Input: part model. Units: mm. Frame: model coordinates. A direction names the side the tool comes from. Coordinates: 2 decimals unless noted, no trailing zeros. Loops run counter-clockwise (first coordinate to the right, second up) from the corner with the lowest first, then second, coordinate; pieces in that order, holes last. Notation, with made-up numbers: (34.25, -23.5) -> (77.25, -23.5) arc R20 ccw to (77.25, 14.5) -> close; hole circle Ø9 at (9.25, -18). An arc over 180 degrees is marked (long way). Put each result on its own line as item: value. Start each with the question number.
1) Cut plane B-B (x = 0). Return the cut outline in (y, z), plus the area to 3 significant figures.
2) Cut plane C-C (y = 1.75). Return the cut outline in (x, z).
3) Cut plane A-A (z = 10). Return the cut outline in (x, y), plus the area to 3 significant figures.
4) Set-up query: faces 1 (the flat face through (2, -4, 20)), 2 (the flat face through (-8, -4, 10)). Return all of +Z, -Z, +X, -X, +Y, -Y with unobstructed straight access to the full face (end or side cutting, diameter ignored); none if empty.
5) Contact query for flat-ended pins moving along their axis: P1, Ø2.5, axis at y = -2, z = 7.5, coming from the +X side; P2, Ø5, axis at x = 0, y = 0, coming from the +Z side; P3, Ø6, axis at x = 14, z = 3, coming from the +Y side; P4, Ø5, axis at y = -1, z = 7, coming from the -X side. Output: stop coordinate, or through.
6) Material intervals for L1, parallel to Y at x = -11.5, z = 2; L2, parallel to Y at x = 0, z = 6.25; L3, parallel to X at y = -2.25, z = 1.5, sorted ascending.
7) Cut plane D-D (z = 4.25). Return the cut outline in (x, y).
8) Pull-direction query (Y, two-part tool) for faces 3 (the flat face through (8, -4, 10)), 4 (the flat face through (13, -8, 12)), 5 (the cylindrical face through (-0.534, 4.065, 9.86)); classes: pulls with the +Y half, pulls with the -Y half, needs draft (parallel to the pull), parting line crosses it, or undercut.
from build123d import *

# Parameters (mm, degrees)
ESBO_O1_R                = 4.1
RESSALTO_EXTRUS_O1_DEPTH = 20
ESBO_O2_R                = 1.6
CORTE_EXTRUS_O1_DEPTH    = 20
FILETE1_R                = 7


with BuildPart() as part:
    # Esboço1 → Ressalto-extrusão1 (new body)
    with BuildSketch(Plane.XY):
        with BuildLine():
            Line((-8, 0), (-8, -8))
            Line((-8, -8), (-18, -8))
            Line((-18, -8), (-18, -12))
            Line((-18, -12), (18, -12))
            Line((18, -12), (18, -8))
            Line((18, -8), (8, -8))
            Line((8, -8), (8, 0))
            ThreePointArc((8, 0), (0, 8), (-8, 0))
        make_face()
        Circle(ESBO_O1_R, mode=Mode.SUBTRACT)
    extrude(amount=RESSALTO_EXTRUS_O1_DEPTH)

    # Esboço2 → Corte-extrusão1 (cut)
    with BuildSketch(Plane(origin=(0, -8, 0), x_dir=(1, 0, 0), z_dir=(0, 1, 0))):
        with Locations(Location((-12.5, -10, 0), (0, 0, 180))):
            Circle(ESBO_O2_R)
        with Locations(Location((12.5, -10, 0), (0, 0, 180))):
            Circle(ESBO_O2_R)
    extrude(amount=-CORTE_EXTRUS_O1_DEPTH, mode=Mode.SUBTRACT)

    # Filete1
    filete1_edges = [part.edges().sort_by_distance(p)[0] for p in [
        (-18, -10, 20),
        (18, -10, 20),
        (18, -10, 0),
        (-18, -10, 0),
    ]]
    fillet(filete1_edges, radius=FILETE1_R)


solid = part.part
Results found:
1. outline: (-12, 0) -> (-4.1, 0) -> (-4.1, 20) -> (-12, 20) -> close; (4.1, 0) -> (8, 0) -> (8, 20) -> (4.1, 20) -> close
1. area: 236 mm2
2. outline: (-7.81, 0) -> (-3.71, 0) -> (-3.71, 20) -> (-7.81, 20) -> close; (3.71, 0) -> (7.81, 0) -> (7.81, 20) -> (3.71, 20) -> close
3. outline: (-18, -12) -> (-14.1, -12) -> (-14.1, -8) -> (-18, -8) -> close; (-10.9, -12) -> (10.9, -12) -> (10.9, -8) -> (8, -8) -> (8, 0) arc R8 ccw to (-8, 0) -> (-8, -8) -> (-10.9, -8) -> close; (14.1, -12) -> (18, -12) -> (18, -8) -> (14.1, -8) -> close; hole circle Ø8.2 at (0, 0)
3. area: 294 mm2
4. face 1: +Z, +X, -X, +Y, -Y
4. face 2: +Z, -Z, -X, +Y
5. P1: stops at x = 8
5. P2: passes through
5. P3: stops at y = -8
5. P4: stops at x = -8
6. L1: y = -12 to -8
6. L2: y = -12 to -4.1, 4.1 to 8
6. L3: x = -8 to -3.43, 3.43 to 8
7. outline: (-17.44, -12) -> (17.44, -12) -> (17.44, -8) -> (8, -8) -> (8, 0) arc R8 ccw to (-8, 0) -> (-8, -8) -> (-17.44, -8) -> close; hole circle Ø8.2 at (0, 0)
8. face 3: needs draft
8. face 4: pulls with the +Y half
8. face 5: undercut
